For this review, take the finished solid that the model builds, in its own axes (mm). Face numbers are marked on the shaded views. A direction names the side the tool comes from. Coordinates: 2 decimals unless noted, no trailing zeros. Order: outer loops, then holes, each group sorted by start corner. A loop starts at its lowest first (then second) coordinate and runs counter-clockwise, first axis right, second up. Notation, with made-up numbers: (50, 24.25) -> (95, 24.25) arc R31 ccw to (95, 50.25) -> close; hole circle Ø1 at (49, 34). An arc over 180 degrees is marked (long way). Answer as a JSON object with one key per item and string values. Group by question number.
1) Wall thickness on L1, parallel to Z at x = 6, y = 5.25; L2, parallel to X at y = 6, z = 1; L3, parallel to Y at x = -10, z = 0: over which ranges is each line inside the solid? List them lowest first.
2) Add section A-A, the plane z = 6.5. Write out the cut boundary in (x, y), then the cut area to 3 significant figures.
3) Add section B-B, the plane y = 1.5. Write out the cut boundary in (x, z).
4) For pin 1 (2.5 mm diameter, centred on x = 9, y = 2.5, fed in from +Z); pin 2 (9 mm diameter, centred on y = 5.5, z = 4, fed in from -X); pin 3 (4 mm diameter, centred on x = 8, z = 3.5, fed in from +Y), all flat-tipped, find the tip position at first contact; note any pin that passes through.
5) Add section D-D, the plane x = -9.5. Write out the cut boundary in (y, z).
6) Machinability: for the marked faces 1, 2 and 3, which of the approach directions +Z, -Z, +X, -X, +Y, -Y give a long, thin tool a straight path to every point of the face, cutting with its end or side? Answer none if there is none.
7) Add section C-C, the plane x = 9.75. Write out the cut boundary in (y, z), then the cut area to 3 significant figures.
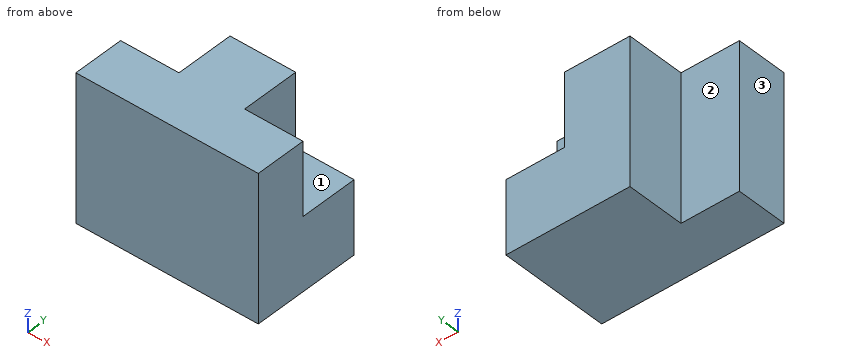
Autodesk Inventor part; units mm, degrees
ref_plane "YZ Plane" through (0, 0, 0) normal (1, 0, 0) x (0, 1, 0)
ref_plane "XZ Plane" through (0, 0, 0) normal (0, 1, 0) x (-1, 0, 0)
ref_plane "XY Plane" through (0, 0, 0) normal (0, 0, 1) x (1, 0, 0)
sketch "草圖1" plane through (0, 0, 0) normal (0, 0, 1) x (1, 0, 0)
  line L0 (-12.5, -7.5) -> (12.5, -7.5)
  line L1 (12.5, -7.5) -> (12.5, 7.5)
  line L2 (12.5, 7.5) -> (-12.5, 7.5)
  line L3 (-12.5, 7.5) -> (-12.5, -7.5)
  line L4 (-12.5, -7.5) -> (12.5, 7.5) construction
  line L5 (12.5, -7.5) -> (-12.5, 7.5) construction
  point P0 (0, 0)
  dimension "d0" = 25
  dimension "d1" = 15
extrude "擠出1" add sketch "草圖1" along normal mid plane 20
sketch "草圖2" plane through (0, 0, 10) normal (0, 0, 1) x (1, 0, 0)
  line L0 (12.5, 7.5) -> (-12.5, 7.5)
  line L1 (-12.5, 7.5) -> (-4.5, 7.5)
  line L2 (-4.5, 7.5) -> (-4.5, -0.5)
  line L3 (-4.5, -0.5) -> (-12.5, -0.5)
  line L4 (-12.5, -0.5) -> (-12.5, 7.5)
  line L5 (12.5, 7.5) -> (4.5, 7.5)
  line L6 (4.5, 7.5) -> (4.5, -0.5)
  line L7 (4.5, -0.5) -> (12.5, -0.5)
  line L8 (12.5, -0.5) -> (12.5, 7.5)
  point P0 (0, 0)
  point P1 (-4.5, 7.5)
  dimension "d4" = 8
  dimension "d5" = 8
  dimension "d6" = 8
extrude "擠出2" cut sketch "草圖2" against normal blind 10 contours L8 L7 L6 L0
extrude "擠出3" cut sketch "草圖2" against normal blind 20 contours L2 L3 L4 L0
properties part number "視圖範例"
Output values:
{
 "1": {"L1": "z = -10 to 0", "L2": "x = -4.5 to 4.5", "L3": "y = -7.5 to -0.5"},
 "2": {"outline": "(-12.5, -7.5) -> (12.5, -7.5) -> (12.5, -0.5) -> (4.5, -0.5) -> (4.5, 7.5) -> (-4.5, 7.5) -> (-4.5, -0.5) -> (-12.5, -0.5) -> close", "area": "247 mm²"},
 "3": {"outline": "(-4.5, -10) -> (12.5, -10) -> (12.5, 0) -> (4.5, 0) -> (4.5, 10) -> (-4.5, 10) -> close"},
 "4": {"pin 1": "stops at z = 0", "pin 2": "stops at x = -4.5", "pin 3": "stops at y = -0.5"},
 "5": {"outline": "(-7.5, -10) -> (-0.5, -10) -> (-0.5, 10) -> (-7.5, 10) -> close"},
 "6": {"face 1": "+Z, +X, +Y", "face 2": "+Z, -Z, -X, +Y", "face 3": "+Z, -Z, -X, +Y, -Y"},
 "7": {"outline": "(-7.5, -10) -> (7.5, -10) -> (7.5, 0) -> (-0.5, 0) -> (-0.5, 10) -> (-7.5, 10) -> close", "area": "220 mm²"}
}
